Build history of the part. All positions in model axes, mm. Face numbers are marked on the shaded views. A direction names the side the tool comes from. Give positions to 0.01 mm unless a question says otherwise; leave off trailing zeros. Loops run counter-clockwise (first coordinate to the right, second up) from the corner with the lowest first, then second, coordinate; pieces in that order, holes last. Notation, with made-up numbers: (45, -7.75) -> (86, -7.75) arc R24 ccw to (86, 29.25) -> close; hole circle Ø8 at (77.5, -36.75). An arc over 180 degrees is marked (long way). Answer as a JSON object with one key per item and string values. Group by question number.
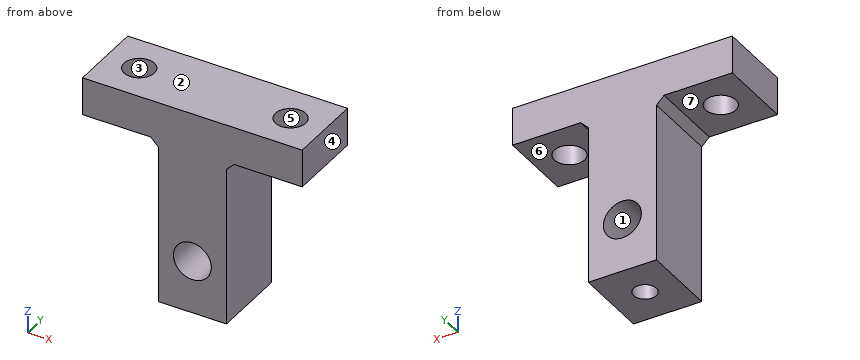
from build123d import *

# Parameters (mm, degrees)
SKETCH1_R           = 2.5
BOSS_EXTRUDE1_DEPTH = 10
SKETCH2_R           = 2
CUT_EXTRUDE1_DEPTH  = 10
SKETCH3_R           = 1.5
CUT_EXTRUDE2_DEPTH  = 4
CHAMFER1_SIZE       = 1


with BuildPart() as part:
    # Sketch1 → Boss-Extrude1 (new body)
    with BuildSketch(Plane(origin=(0, 0, 0), x_dir=(1, 0, 0), z_dir=(0, 1, 0))):
        Polygon((-1.577591036, 0), (-16.077591036, 0), (-16.077591036, 5), (-6.077591036, 5), (-6.077591036, 27), (2.922408964, 27), (2.922408964, 5), (12.922408964, 5), (12.922408964, 0), align=None)
        with Locations((-1.577591036, 20)):
            Circle(SKETCH1_R, mode=Mode.SUBTRACT)
    extrude(amount=BOSS_EXTRUDE1_DEPTH)

    # Sketch2 → Cut-Extrude1 (cut)
    with BuildSketch(Plane.XY):
        with Locations((-11.577591036, 5)):
            Circle(SKETCH2_R)
        with Locations((8.422408964, 4.9503422)):
            Circle(SKETCH2_R)
    extrude(amount=-CUT_EXTRUDE1_DEPTH, mode=Mode.SUBTRACT)

    # Sketch3 → Cut-Extrude2 (cut)
    with BuildSketch(Plane(origin=(0, 0, -27), x_dir=(-1, 0, 0), z_dir=(0, 0, -1))):
        with Locations((1.577591036, 5)):
            Circle(SKETCH3_R)
    extrude(amount=-CUT_EXTRUDE2_DEPTH, mode=Mode.SUBTRACT)

    # Chamfer1
    chamfer1_edges = [part.edges().sort_by_distance(p)[0] for p in [
        (-6.077591036, 5, -5),
        (2.922408964, 5, -5),
    ]]
    chamfer(chamfer1_edges, length=CHAMFER1_SIZE)


solid = part.part
(1) Probe line 1 along X through (y, z) = (3.5, -3.75); line 2 along X through (y, z) = (6, -20); line 3 along X through (y, z) = (7, -15). List the from-to ranges inside material, lowest first. Write a range as [from, to].
(2) Saw through at C-C on x = 7.25. List the corners of the cut face in (y, z).
(3) Pin check, flat tips, straight feed: pin 1 (2.5 mm diameter, centred on x = -1.58, y = 5, fed in from -Z); pin 2 (3 mm diameter, centred on x = -10, y = 6.5, fed in from -Z); pin 3 (1 mm diameter, centred on y = 2.5, z = -21.5, fed in from -X). Stop position of each tip, or through.
(4) 3-axis set-ups, long thin cutter, end or side, ignore diameter. For the marked faces 5, 6 and 7: which of +Z, -Z, +X, -X, +Y, -Y reach the whole face in a straight line?
(5) Pull direction X, two halves, no side cores. Call the marked faces 1, 2, 3 and 4: pulls with the +X half, pulls with the -X half, needs draft (parallel to the pull), parting line crosses it, or undercut.
(6) Saw through at D-D on z = -8. List the corners of the cut face in (x, y), plus the area to 3 significant figures.
(7) Saw through at B-B on z = -20. List the corners of the cut face in (x, y), plus the area to 3 significant figures.
(8) Saw through at A-A on y = 4.25. List the corners of the cut face in (x, z), plus the area to 3 significant figures.
Calculated:
{
 "1": {"line 1": "x = [-16.08, -12.9], [-10.25, 7.05], [9.8, 12.92]", "line 2": "x = [-6.08, -4.08], [0.92, 2.92]", "line 3": "x = [-6.08, 2.92]"},
 "2": {"outline": "(0, -5) -> (3.33, -5) -> (3.33, 0) -> (0, 0) -> close; (6.57, -5) -> (10, -5) -> (10, 0) -> (6.57, 0) -> close"},
 "3": {"pin 1": "stops at z = -23", "pin 2": "stops at z = -5", "pin 3": "stops at x = -6.08"},
 "4": {"face 5": "+Z, -Z", "face 6": "-Z, +X, +Y, -Y", "face 7": "-Z, -X, +Y, -Y"},
 "5": {"face 1": "undercut", "face 2": "needs draft", "face 3": "undercut", "face 4": "pulls with the +X half"},
 "6": {"outline": "(-6.08, 0) -> (2.92, 0) -> (2.92, 10) -> (-6.08, 10) -> close", "area": "90.0 mm^2"},
 "7": {"outline": "(-6.08, 0) -> (-4.08, 0) -> (-4.08, 10) -> (-6.08, 10) -> close; (0.92, 0) -> (2.92, 0) -> (2.92, 10) -> (0.92, 10) -> close", "area": "40.0 mm^2"},
 "8": {"outline": "(-16.08, -5) -> (-13.43, -5) -> (-13.43, 0) -> (-16.08, 0) -> close; (-9.72, -5) -> (-7.08, -5) -> (-6.08, -6) -> (-6.08, -27) -> (-2.88, -27) -> (-2.88, -23) -> (-0.28, -23) -> (-0.28, -27) -> (2.92, -27) -> (2.92, -6) -> (3.92, -5) -> (6.55, -5) -> (6.55, 0) -> (-9.72, 0) -> close; (10.3, -5) -> (12.92, -5) -> (12.92, 0) -> (10.3, 0) -> close; hole circle Ø5 at (-1.58, -20)", "area": "277 mm^2"}
}
